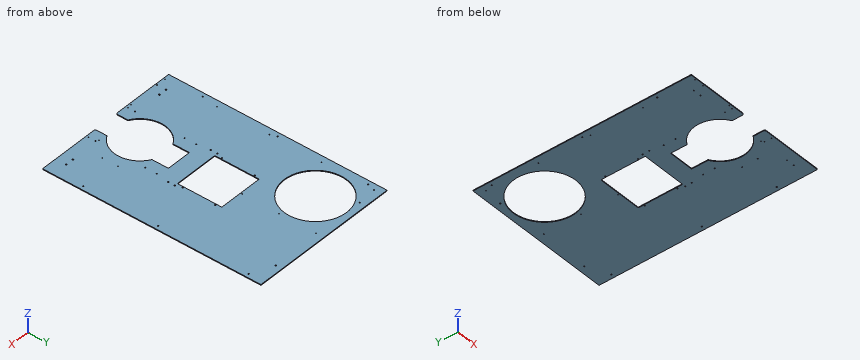
```python
from build123d import *

# Parameters (mm, degrees)
SKETCH1_W                                     = 1219.2
SKETCH1_H                                     = 1778
SKETCH1_R                                     = 254
SKETCH1_W_2                                   = 361.95
SKETCH1_H_2                                   = 361.95
BOSS_EXTRUDE1_DEPTH                           = 6.35
SKETCH3_R                                     = 209.55
CUT_EXTRUDE2_DEPTH                            = 2156.869421486
SKETCH2_W                                     = 203.2
SKETCH2_H                                     = 165.1
CUT_EXTRUDE1_DEPTH                            = 2156.869421486
SKETCH4_R                                     = 3.3655
CUT_EXTRUDE3_DEPTH                            = 2156.869421486
LPATTERN1_COUNT                               = 5
LPATTERN1_PITCH                               = 425.45
SKETCH5_R                                     = 3.429
CUT_EXTRUDE4_DEPTH                            = 2156.869421486
LPATTERN2_COUNT                               = 3
LPATTERN2_PITCH                               = 301.625
SKETCH6_R                                     = 3.3782
CUT_EXTRUDE5_DEPTH                            = 2156.869421486
SKETCH7_R                                     = 3.3782
CUT_EXTRUDE6_DEPTH                            = 2156.869421486
CSK_FOR_1_4_FLAT_HEAD_MACHINE_SCREW1_AT_COUNT = 2
CSK_FOR_1_4_FLAT_HEAD_MACHINE_SCREW1_AT_PITCH = 63.5
LPATTERN3_COUNT                               = 2
LPATTERN3_PITCH                               = 901.7
SKETCH12_R                                    = 4.7625
CUT_EXTRUDE7_DEPTH                            = 2156.869421486
SKETCH14_R                                    = 4.7625
CUT_EXTRUDE8_DEPTH                            = 2156.869421486
SKETCH15_R                                    = 4.7625
CUT_EXTRUDE9_DEPTH                            = 2156.869421486
SKETCH16_R                                    = 4.7625
CUT_EXTRUDE10_DEPTH                           = 2156.869421486
FILLET1_R                                     = 12.7
FILLET2_R                                     = 6.35
SKETCH17_R                                    = 3.937
CUT_EXTRUDE11_DEPTH                           = 2156.869421486
SKETCH18_R                                    = 3.96875
CUT_EXTRUDE12_DEPTH                           = 2156.869421486


with BuildPart() as part:
    # Sketch1 → Boss-Extrude1 (new body)
    with BuildSketch(Plane.XY):
        with Locations((609.6, 889)):
            Rectangle(SKETCH1_W, SKETCH1_H)
        with Locations((330.2, 1473.2)):
            Circle(SKETCH1_R, mode=Mode.SUBTRACT)
        with Locations((609.6, 917.575)):
            Rectangle(SKETCH1_W_2, SKETCH1_H_2, mode=Mode.SUBTRACT)
    extrude(amount=BOSS_EXTRUDE1_DEPTH)

    # Sketch3 → Cut-Extrude2 (cut, through all)
    with BuildSketch(Plane.XY.offset(6.35)):
        with Locations((609.6, 279.4)):
            Circle(SKETCH3_R)
    extrude(amount=-CUT_EXTRUDE2_DEPTH, mode=Mode.SUBTRACT)

    # Sketch2 → Cut-Extrude1 (cut, through all)
    with BuildSketch(Plane.XY.offset(6.35)):
        with Locations((609.6, 44.45)):
            Rectangle(SKETCH2_W, SKETCH2_H)
        with Locations((609.6, 514.35)):
            Rectangle(SKETCH2_W, SKETCH2_H)
    extrude(amount=-CUT_EXTRUDE1_DEPTH, mode=Mode.SUBTRACT)

    # Sketch4 → Cut-Extrude3 (cut, through all)
    with BuildSketch(Plane.XY.offset(6.35)):
        with Locations((50.8, 12.7)):
            Circle(SKETCH4_R)
    cut_extrude3 = extrude(amount=-CUT_EXTRUDE3_DEPTH, mode=Mode.SUBTRACT)

    # LPattern1: Cut-Extrude3 ×5
    with Locations(*[(0, i * LPATTERN1_PITCH, 0) for i in range(1, LPATTERN1_COUNT)]):
        add(cut_extrude3, mode=Mode.SUBTRACT)

    # Sketch5 → Cut-Extrude4 (cut, through all)
    with BuildSketch(Plane.XY.offset(6.35)):
        with Locations((609.6, 1714.5)):
            Circle(SKETCH5_R)
    cut_extrude4 = extrude(amount=-CUT_EXTRUDE4_DEPTH, mode=Mode.SUBTRACT)

    # LPattern2: Cut-Extrude4 ×3
    with Locations(*[(0, -i * LPATTERN2_PITCH, 0) for i in range(1, LPATTERN2_COUNT)]):
        add(cut_extrude4, mode=Mode.SUBTRACT)

    # Sketch6 → Cut-Extrude5 (cut, through all)
    with BuildSketch(Plane.XY.offset(6.35)):
        with Locations((127, 12.7)):
            Circle(SKETCH6_R)
        with Locations((381, 12.7)):
            Circle(SKETCH6_R)
    extrude(amount=-CUT_EXTRUDE5_DEPTH, mode=Mode.SUBTRACT)

    # Sketch7 → Cut-Extrude6 (cut, through all)
    with BuildSketch(Plane.XY.offset(6.35)):
        with Locations((777.605208253, 88.9)):
            Circle(SKETCH7_R)
        with Locations((898.525, 342.9)):
            Circle(SKETCH7_R)
        with Locations((898.525, 215.9)):
            Circle(SKETCH7_R)
    extrude(amount=-CUT_EXTRUDE6_DEPTH, mode=Mode.SUBTRACT)

    # Sketch11 → CSK for 1/4 Flat Head Machine Screw1 (revolve, cut)
    with BuildSketch(Plane(origin=(127, 85.725, 6.35), x_dir=(0, -1, 0), z_dir=(1, 0, 0))):
        Polygon((0, 0), (0, 6.35), (3.57124, 6.35), (3.57124, 3.298865467), (6.4389, 0), align=None)
    csk_for_1_4_flat_head_machine_screw1 = revolve(axis=Axis((127, 85.725, 12.7), (0, 0, -1)), mode=Mode.SUBTRACT)

    # CSK for 1/4 Flat Head Machine Screw1 at: CSK for 1/4 Flat Head Machine Screw1 ×2
    with Locations(*[(i * CSK_FOR_1_4_FLAT_HEAD_MACHINE_SCREW1_AT_PITCH, 0, 0) for i in range(1, CSK_FOR_1_4_FLAT_HEAD_MACHINE_SCREW1_AT_COUNT)]):
        add(csk_for_1_4_flat_head_machine_screw1, mode=Mode.SUBTRACT)

    # LPattern3: CSK for 1/4 Flat Head Machine Screw1 ×2
    with Locations(*[(i * LPATTERN3_PITCH, 0, 0) for i in range(1, LPATTERN3_COUNT)]):
        add(csk_for_1_4_flat_head_machine_screw1, mode=Mode.SUBTRACT)

    # LPattern3 copy 1 sketch → LPattern3 copy 1 (revolve, cut)
    with BuildSketch(Plane(origin=(1092.2, 85.725, 6.35), x_dir=(0, -1, 0), z_dir=(1, 0, 0))):
        Polygon((0, 0), (0, 6.35), (3.57124, 6.35), (3.57124, 3.298865467), (6.4389, 0), align=None)
    revolve(axis=Axis((1092.2, 85.725, 12.7), (0, 0, -1)), mode=Mode.SUBTRACT)

    # Sketch12 → Cut-Extrude7 (cut, through all)
    with BuildSketch(Plane.XY.offset(6.35)):
        with Locations((203.2, 1727.2)):
            Circle(SKETCH12_R)
        with Locations((1016, 1727.2)):
            Circle(SKETCH12_R)
    extrude(amount=-CUT_EXTRUDE7_DEPTH, mode=Mode.SUBTRACT)

    # Sketch14 → Cut-Extrude8 (cut, through all)
    with BuildSketch(Plane.XY.offset(6.35)):
        with Locations((31.75, 1651)):
            Circle(SKETCH14_R)
        with Locations((31.75, 914.4)):
            Circle(SKETCH14_R)
        with Locations((31.75, 304.8)):
            Circle(SKETCH14_R)
    cut_extrude8 = extrude(amount=-CUT_EXTRUDE8_DEPTH, mode=Mode.SUBTRACT)

    # Mirror1: Cut-Extrude8 across plane
    add(cut_extrude8.mirror(Plane.ZY.offset(-609.6)), mode=Mode.SUBTRACT)

    # Sketch15 → Cut-Extrude9 (cut, through all)
    with BuildSketch(Plane.XY.offset(6.35)):
        with Locations((403.225, 736.6)):
            Circle(SKETCH15_R)
        with Locations((403.225, 682.625)):
            Circle(SKETCH15_R)
    cut_extrude9 = extrude(amount=-CUT_EXTRUDE9_DEPTH, mode=Mode.SUBTRACT)

    # Mirror2: Cut-Extrude9 across plane
    add(cut_extrude9.mirror(Plane.ZY.offset(-609.6)), mode=Mode.SUBTRACT)

    # Sketch16 → Cut-Extrude10 (cut, through all)
    with BuildSketch(Plane.XY.offset(6.35)):
        with Locations((419.1, 1054.1)):
            Circle(SKETCH16_R)
        with Locations((419.1, 787.4)):
            Circle(SKETCH16_R)
        with Locations((800.1, 1054.1)):
            Circle(SKETCH16_R)
        with Locations((800.1, 787.4)):
            Circle(SKETCH16_R)
    extrude(amount=-CUT_EXTRUDE10_DEPTH, mode=Mode.SUBTRACT)

    # Fillet1
    fillet1_edges = [part.edges().sort_by_distance(p)[0] for p in [
        (508, 0, 3.175),
        (711.2, 0, 3.175),
    ]]
    fillet(fillet1_edges, radius=FILLET1_R)

    # Fillet2
    fillet2_edges = [part.edges().sort_by_distance(p)[0] for p in [
        (428.625, 1098.55, 3.175),
        (428.625, 736.6, 3.175),
        (790.575, 736.6, 3.175),
        (790.575, 1098.55, 3.175),
        (711.2, 596.9, 3.175),
        (508, 596.9, 3.175),
        (0, 0, 3.175),
        (1219.2, 0, 3.175),
    ]]
    fillet(fillet2_edges, radius=FILLET2_R)

    # Sketch17 → Cut-Extrude11 (cut, through all)
    with BuildSketch(Plane.XY.offset(6.35)):
        with Locations((416.56762, 76.2)):
            Circle(SKETCH17_R)
        with Locations((416.56762, 19.05)):
            Circle(SKETCH17_R)
        with Locations((797.56762, 19.05)):
            Circle(SKETCH17_R)
        with Locations((797.56762, 76.2)):
            Circle(SKETCH17_R)
    extrude(amount=-CUT_EXTRUDE11_DEPTH, mode=Mode.SUBTRACT)

    # Sketch18 → Cut-Extrude12 (cut, through all)
    with BuildSketch(Plane.XY.offset(6.35)):
        with Locations((418.15512, 576.972045059)):
            Circle(SKETCH18_R)
        with Locations((418.15512, 481.722045059)):
            Circle(SKETCH18_R)
        with Locations((799.15512, 481.722045059)):
            Circle(SKETCH18_R)
        with Locations((799.15512, 576.972045059)):
            Circle(SKETCH18_R)
    extrude(amount=-CUT_EXTRUDE12_DEPTH, mode=Mode.SUBTRACT)


solid = part.part
```
Check sheet for the modelled part. Datum: model origin and axes. Units: mm. Give positions to 0.01 mm unless a question says otherwise; leave off trailing zeros. Order: outer loops, then holes, each group sorted by start corner. A loop starts at its lowest first (then second) coordinate and runs counter-clockwise, first axis right, second up. Notation, with made-up numbers: (29.25, -35.75) -> (74.25, -35.75) arc R13 ccw to (74.25, -13.75) -> close; hole circle Ø2 at (-13, -31.5). An arc over 180 degrees is marked (long way). Return JSON: item names as keys, results as strings.
1. Go/stop test with flat-tipped pins: P1, Ø8, axis at x = 127, y = 85.725, coming from the +Z side; P2, Ø3, axis at x = 633, z = 3, coming from the -Y side; P3, Ø5.5, axis at x = 50.8, y = 438.15, coming from the -Z side. Record where each tip stops, or that it passes through.
From the geometry:
{"P1": "z = 3.54", "P2": "y = 596.9", "P3": "through"}
2. Material ranges on probe 1 along Y at (x, z) = (428, 4.75); probe 2 along X at (y, z) = (281, 3.75); probe 3 along Y at (x, z) = (381.5, 0.5), recorded low to high. Write a range as [from, to].
From the geometry:
{"probe 1": "[0, 174.84], [383.96, 1238.78], [1707.62, 1778]", "probe 2": "[0, 400.06], [819.14, 1219.2]", "probe 3": "[0, 9.36], [16.04, 1224.43], [1721.97, 1778]"}
3. Cross-section at D-D, the plane z = 1. Count the separate pieces of the cut face and the enclosed holes in it, plus the area to 3 significant figures.
From the geometry:
{"separate pieces": "1", "enclosed holes": "43", "area": "1,650,000 mm^2"}
4. Cross-section at A-A, the plane y = 974. Record the cut outline in (x, z) (3 decimals), plus the area to 3 significant figures.
From the geometry:
{"outline": "(0, 0) -> (428.625, 0) -> (428.625, 6.35) -> (0, 6.35) -> close; (790.575, 0) -> (1219.2, 0) -> (1219.2, 6.35) -> (790.575, 6.35) -> close", "area": "5,440 mm^2"}
5. Cross-section at C-C, the plane x = 748. Record the cut outline in (y, z), plus the area to 3 significant figures.
From the geometry:
{"outline": "(0, 0) -> (122.06, 0) -> (122.06, 6.35) -> (0, 6.35) -> close; (436.74, 0) -> (736.6, 0) -> (736.6, 6.35) -> (436.74, 6.35) -> close; (1098.55, 0) -> (1778, 0) -> (1778, 6.35) -> (1098.55, 6.35) -> close", "area": "6,990 mm^2"}
6. Cross-section at B-B, the plane x = 295. Record the cut outline in (y, z).
From the geometry:
{"outline": "(0, 0) -> (1221.65, 0) -> (1221.65, 6.35) -> (0, 6.35) -> close; (1724.75, 0) -> (1778, 0) -> (1778, 6.35) -> (1724.75, 6.35) -> close"}
